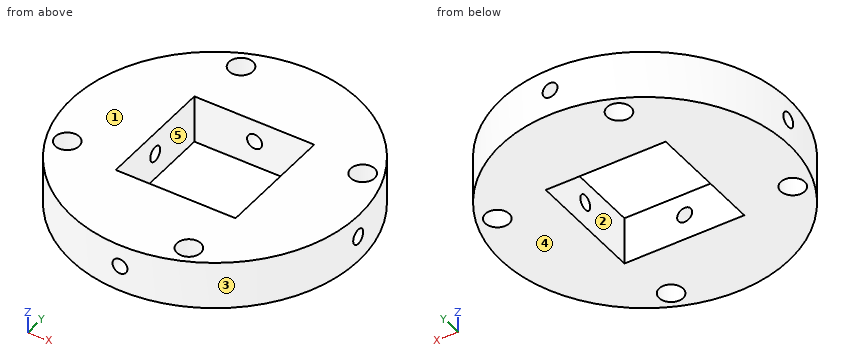
from build123d import *

# Parameters (mm, degrees)
SKETCH1_R           = 7.62
BOSS_EXTRUDE1_DEPTH = 2.54
SKETCH2_W           = 6.35
SKETCH2_H           = 6.35
CUT_EXTRUDE1_DEPTH  = 12.071603317
SKETCH3_R           = 0.635
CUT_EXTRUDE2_DEPTH  = 12.071603317
CIRPATTERN1_COUNT   = 4
CIRPATTERN2_COUNT   = 4


with BuildPart() as part:
    # Sketch1 → Boss-Extrude1 (new body)
    with BuildSketch(Plane.XY):
        Circle(SKETCH1_R)
    extrude(amount=BOSS_EXTRUDE1_DEPTH)

    # Sketch2 → Cut-Extrude1 (cut, through all)
    with BuildSketch(Plane.XY.offset(2.54)):
        Rectangle(SKETCH2_W, SKETCH2_H)
    extrude(amount=-CUT_EXTRUDE1_DEPTH, mode=Mode.SUBTRACT)

    # Sketch3 → Cut-Extrude2 (cut, through all)
    with BuildSketch(Plane.XY.offset(2.54)):
        with Locations((-2.622739109, 6.103536802)):
            Circle(SKETCH3_R)
    cut_extrude2 = extrude(amount=-CUT_EXTRUDE2_DEPTH, mode=Mode.SUBTRACT)

    # CirPattern1: Cut-Extrude2 ×4 about axis
    cirpattern1_axis = Axis((0, 0, 0), (0, 0, 1))
    for i in range(1, CIRPATTERN1_COUNT):
        add(cut_extrude2.rotate(cirpattern1_axis, i * 360 / CIRPATTERN1_COUNT), mode=Mode.SUBTRACT)

    # Sketch6 → 1/32 (0.03125) Diameter Hole1 (revolve, cut)
    with BuildSketch(Plane(origin=(0.038702284, 7.619901714, 1.36675571), x_dir=(-0.9999871015937097, 0.005079039890736663, 0), z_dir=(0, 0, 1))):
        Polygon((0, 0), (0, 6.683017666), (0.396875, 6.35), (0.396875, 0), align=None)
    f_1_32_0_03125_diameter_hole1 = revolve(axis=Axis((0.070954187, 13.969819809, 1.36675571), (-0.005079039890736664, -0.9999871015937097, 0)), mode=Mode.SUBTRACT)

    # CirPattern2: 1/32 (0.03125) Diameter Hole1 ×4 about axis
    cirpattern2_axis = Axis((0, 0, 2.54), (0, 0, -1))
    for i in range(1, CIRPATTERN2_COUNT):
        add(f_1_32_0_03125_diameter_hole1.rotate(cirpattern2_axis, i * 360 / CIRPATTERN2_COUNT), mode=Mode.SUBTRACT)


solid = part.part
Can you work these out from the model? Positions are in its coordinate system, mm. Face numbers are marked on the shaded views. A direction names the side the tool comes from. Coordinates: 2 decimals unless noted, no trailing zeros. Write each loop counter-clockwise with the first axis right and the second up, starting at its lowest first coordinate (ties: lowest second). Pieces come first, ordered by that corner, then holes. Notation, with made-up numbers: (-13, 74) - (37, 74) arc R18 ccw to (37, 103) - close; hole circle Ø4 at (88.5, 24.25). An arc over 180 degrees is marked (long way). Return JSON: item names as keys, results as strings. Group by question number.
Item 1: If we section it at C-C (x = 0): Count the separate pieces of the cut face and the enclosed holes in it, then the cut area to 3 significant figures.
Item 2: Please list where these lines run through material, in increasing order: probe 1 along Z at (x, y) = (0, -4); probe 2 along Y at (x, z) = (-2.75, 0.55) (3 decimals); probe 3 along Y at (x, z) = (-2.5, 1.8) (3 decimals).
Item 3: I'm going to push a flat-ended pin straight in: pin 1 Ø1.3 at (y, z) = (-1, 1.5) entering from +X. Where does the tip first touch, or does it pass through?
Item 4: Which directions (+Z, -Z, +X, -X, +Y, -Y) give clear straight access to the entire face, cutting with the end or side of a thin tool? Please do the marked faces 1 and 2.
Item 5: We'd pull the mould along X, two halves only. Please class the marked faces 3, 4 and 5: pulls with the +X half, pulls with the -X half, needs draft (parallel to the pull), parting line crosses it, or undercut.
Item 6: If we section it at A-A (z = 0.35): Write out the boundary of the cut face in (x, y) (3 decimals).
Item 7: If we section it at B-B (y = 2.25): Write out the boundary of the cut face in (x, z) (3 decimals), then the cut area to 3 significant figures.
Return value:
{
 "1": {"separate pieces": "4", "enclosed holes": "0", "area": "15.5 mm^2"},
 "2": {"probe 1": "z = 0 to 0.97, 1.76 to 2.54", "probe 2": "y = -7.106 to -3.175, 3.175 to 5.481, 6.726 to 7.106", "probe 3": "y = -7.198 to -3.175, 3.175 to 5.481, 6.727 to 7.198"},
 "3": {"pin 1": "stops at x = 7.61"},
 "4": {"face 1": "+Z, +X, -X, +Y, -Y", "face 2": "+Z, -Z"},
 "5": {"face 3": "parting line crosses it", "face 4": "needs draft", "face 5": "undercut"},
 "6": {"outline": "circle Ø15.24 at (0, 0); hole circle Ø1.27 at (-6.104, -2.623); hole circle Ø1.27 at (-2.623, 6.104); hole (-3.175, -3.175) - (3.175, -3.175) - (3.175, 3.175) - (-3.175, 3.175) - close; hole circle Ø1.27 at (2.623, -6.104); hole circle Ø1.27 at (6.104, 2.623)"},
 "7": {"outline": "(-7.28, 0) - (-3.175, 0) - (-3.175, 2.54) - (-7.28, 2.54) - close; (3.175, 0) - (5.589, 0) - (5.589, 2.54) - (3.175, 2.54) - close; (6.618, 0) - (7.28, 0) - (7.28, 2.54) - (6.618, 2.54) - close", "area": "18.2 mm^2"}
}
